Part model, mm, in its own coordinate system. Face numbers are marked on the shaded views. A direction names the side the tool comes from. Round coordinates to 2 decimals unless told otherwise and drop trailing zeros. Write each loop counter-clockwise with the first axis right and the second up, starting at its lowest first coordinate (ties: lowest second). Pieces come first, ordered by that corner, then holes. Notation, with made-up numbers: (-9.5, -31) -> (-5.5, -31) arc R31 ccw to (-5.5, -1) -> close; hole circle Ø11 at (62.25, -26). An arc over 180 degrees is marked (long way). Use CSV: the item, a comma, the result in double quotes. Start each with the question number.
```python
from build123d import *

# Parameters (mm, degrees)
SKETCH1_W           = 42
SKETCH1_H           = 32.004
BOSS_EXTRUDE1_DEPTH = 3.175
SKETCH2_W           = 42
SKETCH2_H           = 32.385
BOSS_EXTRUDE2_DEPTH = 3.175
SKETCH3_R           = 10.9982
SKETCH3_R_2         = 1.4224
CUT_EXTRUDE1_DEPTH  = 5.08
SKETCH4_R           = 4.0005
SKETCH4_R_2         = 1.8288
CUT_EXTRUDE2_DEPTH  = 5.1054
CUT_EXTRUDE3_DEPTH  = 40.373698125


with BuildPart() as part:
    # Sketch1 → Boss-Extrude1 (new body)
    with BuildSketch(Plane(origin=(0, 0, 0), x_dir=(1, 0, 0), z_dir=(0, 1, 0))):
        Rectangle(SKETCH1_W, SKETCH1_H)
    extrude(amount=BOSS_EXTRUDE1_DEPTH)

    # Sketch2 → Boss-Extrude2 (add)
    with BuildSketch(Plane(origin=(0, 0, -16.002), x_dir=(-1, 0, 0), z_dir=(0, 0, -1))):
        with Locations((0, 16.1925)):
            Rectangle(SKETCH2_W, SKETCH2_H)
    extrude(amount=-BOSS_EXTRUDE2_DEPTH)

    # Sketch3 → Cut-Extrude1 (cut)
    with BuildSketch(Plane.XY.offset(-12.827)):
        with Locations((-0.665996173, 10.8585)):
            Circle(SKETCH3_R)
        with Locations((-16.172696173, 26.3652)):
            Circle(SKETCH3_R_2)
        with Locations((14.840703827, 26.3652)):
            Circle(SKETCH3_R_2)
    extrude(amount=-CUT_EXTRUDE1_DEPTH, mode=Mode.SUBTRACT)

    # Sketch4 → Cut-Extrude2 (cut)
    with BuildSketch(Plane(origin=(0, 3.175, 0), x_dir=(1, 0, 0), z_dir=(0, 1, 0))):
        with Locations(Location((-10.14648729, -6.038137545, 0), (0, 0, 270))):
            Circle(SKETCH4_R)
        with Locations(Location((15.27051293, -11.541044372, 0), (0, 0, 270))):
            Circle(SKETCH4_R_2)
        with Locations(Location((15.27051293, 2.545639175, 0), (0, 0, 270))):
            Circle(SKETCH4_R_2)
    extrude(amount=-CUT_EXTRUDE2_DEPTH, mode=Mode.SUBTRACT)

    # Sketch5 → Cut-Extrude3 (cut, through all)
    with BuildSketch(Plane(origin=(0, 3.175, 0), x_dir=(1, 0, 0), z_dir=(0, 1, 0))):
        Polygon((-16.015261935, -16.002), (-21, -11.017261935), (-21, -16.002), align=None)
    extrude(amount=-CUT_EXTRUDE3_DEPTH, mode=Mode.SUBTRACT)


solid = part.part
```
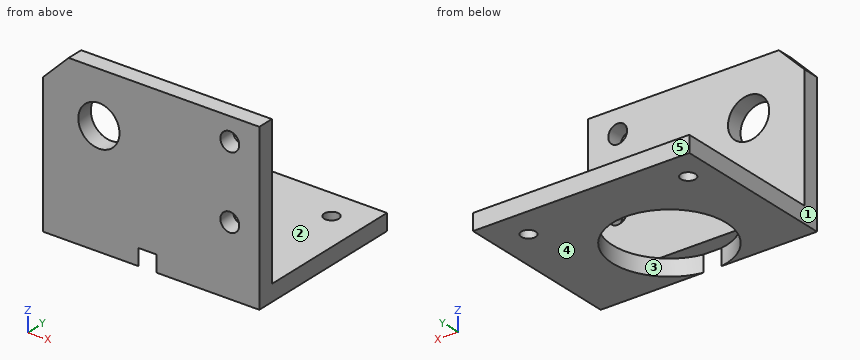
1. Which spindle directions (+Z, -Z, +X, -X, +Y, -Y) get a long thin tool onto all of the face, cutting with end or side? Do the marked faces 1 and 2. Say none if no direction does.
2. Drill centre lines: line 1 along Z through (x, y) = (2.5, 3); line 2 along Z through (x, y) = (14, 16); line 3 along Y through (x, z) = (-17, 6) (3 decimals). Where is each one in solid material? Low to high. Write a range as [from, to].
3. Pull direction Y, two halves, no side cores. Call the marked faces 3, 4 and 5: released by +Y, released by -Y, zero draft, split by the parting line, or undercut.
4. Band-saw the part on A-A (y = 9). List the corners of the cut face in (x, z).
5. Band-saw the part on B-B (x = -13.5). List the corners of the cut face in (y, z) (3 decimals), then the cut area to 3 significant figures.
6. Band-saw the part on C-C (x = -7). List the corners of the cut face in (y, z) (3 decimals), then the cut area to 3 significant figures.
7. Band-saw the part on D-D (z = -6.5). List the corners of the cut face in (x, y) (3 decimals).
8. Flat gauge pins, fed straight in: pin 1 (2.5 mm diameter, centred on x = -1, y = 2.5, fed in from -Z); pin 2 (1 mm diameter, centred on x = 5.5, y = 28, fed in from +Z); pin 3 (8.5 mm diameter, centred on x = 0.5, z = -2, fed in from +Y) (3 decimals). Where does each tip first touch, or does it go through?
Answers below:
1,face 1,"+Z, -Z, -X, +Y, -Y"
1,face 2,"+Z, +X, -X, +Y"
2,line 1,"z = [-12.83, 16]"
2,line 2,"z = [-16, -12.83]"
2,line 3,"y = [0, 3.175]"
3,face 3,"undercut"
3,face 4,"zero draft"
3,face 5,"released by +Y"
4,outline,"(-21, -16) -> (-11.51, -16) -> (-11.51, -12.83) -> (-21, -12.83) -> close; (10.17, -16) -> (21, -16) -> (21, -12.83) -> (10.17, -12.83) -> close"
5,outline,"(0, -16.002) -> (32.385, -16.002) -> (32.385, -12.827) -> (3.175, -12.827) -> (3.175, 3.857) -> (0, 3.857) -> close; (0, 8.219) -> (3.175, 8.219) -> (3.175, 16.002) -> (0, 16.002) -> close"
5,area,"181 mm^2"
6,outline,"(0, -16.002) -> (1.867, -16.002) -> (1.867, -12.827) -> (3.175, -12.827) -> (3.175, 3.568) -> (0, 3.568) -> close; (0, 8.509) -> (3.175, 8.509) -> (3.175, 16.002) -> (0, 16.002) -> close; (19.85, -16.002) -> (32.385, -16.002) -> (32.385, -12.827) -> (19.85, -12.827) -> close"
6,area,"122 mm^2"
7,outline,"(-21, 0) -> (21, 0) -> (21, 3.175) -> (-21, 3.175) -> close"
8,pin 1,"stops at z = -12.83"
8,pin 2,"stops at z = -12.83"
8,pin 3,"stops at y = 3.175"
